```python
from build123d import *

# Parameters (mm, degrees)
SKETCH_1_W               = 5.5
SKETCH_1_H               = 25
CUT_EXTRUDE_1_DEPTH      = 27.182054923
CUT_EXTRUDE_1_DEPTH_BACK = 27.182054923
SKETCH_3_R               = 3.1
SKETCH_4_R               = 4
CUT_EXTRUDE_2_DEPTH      = 24


with BuildPart() as part:
    # 草图1 → 旋转1 (revolve)
    with BuildSketch(Plane.XY, mode=Mode.PRIVATE) as revolve_1_sk:
        with Locations((2.75, 12.5)):
            Rectangle(SKETCH_1_W, SKETCH_1_H)
    revolve(revolve_1_sk.sketch.rotate(Axis((0, 25, 0), (0, 1, 0)), 180), axis=Axis((0, 25, 0), (0, 1, 0)))

    # 草图3 → 切除-拉伸1 (cut, two sides: drawn at the far end of the back side and taken through both)
    with BuildSketch(Plane.XY.offset(-CUT_EXTRUDE_1_DEPTH_BACK)):
        with Locations((0, 17.3)):
            Circle(SKETCH_3_R)
    extrude(amount=CUT_EXTRUDE_1_DEPTH + CUT_EXTRUDE_1_DEPTH_BACK, mode=Mode.SUBTRACT)

    # 草图4 → 切除-拉伸2 (cut)
    with BuildSketch(Plane.XZ):
        Circle(SKETCH_4_R)
    extrude(amount=-CUT_EXTRUDE_2_DEPTH, mode=Mode.SUBTRACT)


solid = part.part
```
Part model, mm, in its own coordinate system. A direction names the side the tool comes from. Coordinates: 2 decimals unless noted, no trailing zeros. Order: outer loops, then holes, each group sorted by start corner. A loop starts at its lowest first (then second) coordinate and runs counter-clockwise, first axis right, second up. Notation, with made-up numbers: (-22, 84) - (-7, 84) arc R29 ccw to (-7, 112) - close; hole circle Ø3 at (22.25, 70). An arc over 180 degrees is marked (long way). Return JSON: item names as keys, results as strings. Group by question number.
Item 1: Cut at C-C (z = 0). List the corners of the cut face in (x, y).
Item 2: Cut at B-B (y = 17.3). List the corners of the cut face in (x, z), plus the area to 3 significant figures.
Item 3: Drill centre lines: probe 1 along Z at (x, y) = (0, 12.75); probe 2 along Y at (x, z) = (-2, -2); probe 3 along X at (y, z) = (17.75, -0.25). Where is each one in solid material? Low to high. Write a range as from..to.
Item 4: Which spindle directions (+Z, -Z, +X, -X, +Y, -Y) get a long thin tool onto all of the face, cutting with end or side? Do faces 4 (the face through (3.695, 11.832, -1.532)), 5 (the face through (-4, 0, -2)). Say none if no direction does.
Item 5: Cut at A-A (x = 0). List the corners of the cut face in (y, z), plus the area to 3 significant figures.
Item 6: Pull direction X, two halves, no side cores. Call faces 1 (the face through (0, 24, 0)), 2 (the face through (0, 25, 0)), 3 (the face through (5.495, 12.675, 0.242)): pulls with the +X half, pulls with the -X half, needs draft (parallel to the pull), parting line crosses it, or undercut.
Item 7: Pin check, flat tips, straight feed: pin 1 (1 mm diameter, centred on x = 1.5, y = 14, fed in from -Z); pin 2 (5 mm diameter, centred on x = -4, y = 16, fed in from +Z); pin 3 (1 mm diameter, centred on x = -3.5, y = 20, fed in from +Z). Stop position of each tip, or through.
Item 8: Cut at D-D (y = 2.25). List the corners of the cut face in (x, z), plus the area to 3 significant figures.
Check values:
{
 "1": {"outline": "(-5.5, 0) - (-4, 0) - (-4, 24) - (4, 24) - (4, 0) - (5.5, 0) - (5.5, 25) - (-5.5, 25) - close"},
 "2": {"outline": "(-3.1, -4.54) - (-3.1, -2.53) arc R4 cw to (-3.1, 2.53) - (-3.1, 4.54) arc R5.5 ccw to start; (3.1, -4.54) arc R5.5 ccw to (3.1, 4.54) - (3.1, 2.53) arc R4 cw to (3.1, -2.53) - close", "area": "24.4 mm2"},
 "3": {"probe 1": "z = -5.5..-4, 4..5.5", "probe 2": "y = 24..25", "probe 3": "x = -5.49..-3.99, 3.99..5.49"},
 "4": {"face 4": "-Y", "face 5": "+Z, -Z, +X, -X, -Y"},
 "5": {"outline": "(0, -5.5) - (14.2, -5.5) - (14.2, -4) - (0, -4) - close; (0, 4) - (14.2, 4) - (14.2, 5.5) - (0, 5.5) - close; (20.4, -5.5) - (25, -5.5) - (25, 5.5) - (20.4, 5.5) - (20.4, 4) - (24, 4) - (24, -4) - (20.4, -4) - close", "area": "64.4 mm2"},
 "6": {"face 1": "undercut", "face 2": "needs draft", "face 3": "parting line crosses it"},
 "7": {"pin 1": "stops at z = -5.41", "pin 2": "stops at z = 5.19", "pin 3": "stops at z = 4.61"},
 "8": {"outline": "circle Ø11 at (0, 0); hole circle Ø8 at (0, 0)", "area": "44.8 mm2"}
}
